Here's how the part is built. I have some questions about the finished solid (model axes, mm). Face numbers are marked on the shaded views. Round coordinates to 2 decimals unless told otherwise and drop trailing zeros. Order: outer loops, then holes, each group sorted by start corner. A loop starts at its lowest first (then second) coordinate and runs counter-clockwise, first axis right, second up. Notation, with made-up numbers: (-29.5, 15) - (-0.5, 15) arc R19 ccw to (-0.5, 25) - close; hole circle Ø10 at (23, 85). An arc over 180 degrees is marked (long way). One line per item, written item: value.
from build123d import *

# Parameters (mm, degrees)
ESQUISSE1_R             = 3.65
ESQUISSE1_R_2           = 2.25
BASE_EXTRUSION_DEPTH    = 1.5
ENL_V_MAT_EXTRU_1_DEPTH = 6.375406961


with BuildPart() as part:
    # Esquisse1 → Base-Extrusion (new body)
    with BuildSketch(Plane.XY):
        Circle(ESQUISSE1_R)
        Circle(ESQUISSE1_R_2, mode=Mode.SUBTRACT)
    extrude(amount=BASE_EXTRUSION_DEPTH)

    # Esquisse2 → Enlèv. mat.-Extru.1 (cut, through all)
    with BuildSketch(Plane(origin=(0, 0, 0), x_dir=(0, 0, -1), z_dir=(1, 0, 0))):
        Polygon((-1.5, -0.154321058), (0, 0.735714302), (0, 0.154321058), (-1.5, -0.735714302), align=None)
    extrude(amount=ENL_V_MAT_EXTRU_1_DEPTH, mode=Mode.SUBTRACT)


solid = part.part
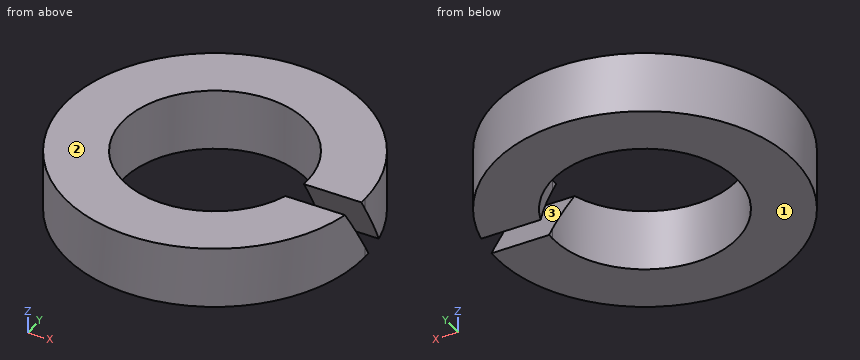
Q1. If I drill on line 1 along Y through (x, z) = (0, 0.45); line 2 along X through (y, z) = (0, 0.9), over which ranges is the centre line in solid material (lowest first)?
Results list:
line 1: -3.65 to -2.25, 2.25 to 3.65
line 2: -3.65 to -2.25
Q2. If we section it at C-C, the plane z = 1: Please give me the cut outline in (x, y).
Results list:
outline: (2.21, -0.44) arc R2.25 cw (long way) to (2.25, 0.14) - (3.65, 0.14) arc R3.65 ccw (long way) to (3.62, -0.44) - close
Q3. We'd pull the mould along Z, two halves only. Please class the marked faces 1, 2 and 3: released by +Z, released by -Z, zero draft, split by the parting line, or undercut.
Results list:
face 1: released by -Z
face 2: released by +Z
face 3: undercut
Q4. If we section it at D-D, the plane x = -2.5: Please give me the cut outline in (y, z), then the cut area to 3 significant figures.
Results list:
outline: (-2.66, 0) - (2.66, 0) - (2.66, 1.5) - (-2.66, 1.5) - close
area: 7.98 mm²
Q5. Will this pin go through, and if not, where does the flat tip stop? pin 1 (1.5 mm diameter, centred on x = -1, y = -1.5, fed in from +Z).
Results list:
pin 1: z = 1.5
Q6. If we section it at A-A, the plane x = 0: Please give me the cut outline in (y, z).
Results list:
outline: (-3.65, 0) - (-2.25, 0) - (-2.25, 1.5) - (-3.65, 1.5) - close; (2.25, 0) - (3.65, 0) - (3.65, 1.5) - (2.25, 1.5) - close
Q7. If we section it at B-B, the plane y = 2: Please give me the cut outline in (x, z).
Results list:
outline: (-3.05, 0) - (-1.03, 0) - (-1.03, 1.5) - (-3.05, 1.5) - close; (1.03, 0) - (3.05, 0) - (3.05, 1.5) - (1.03, 1.5) - close
